```python
from build123d import *

# Parameters (mm, degrees)
SKETCH1_W           = 24.54
SKETCH1_H           = 35.2
MAIN_BODY_DEPTH     = 35.2
SKETCH2_R           = 11
LIP_DEPTH           = 2.25
SKETCH3_R           = 2.5
SHAFT_DEPTH         = 14
CHAMFER1_SIZE       = 5
SKETCH4_R           = 1.5
BOSS_EXTRUDE4_DEPTH = 6


with BuildPart() as part:
    # Sketch1 → Main body (new body)
    with BuildSketch(Plane(origin=(0, 0, 0), x_dir=(1, 0, 0), z_dir=(0, 1, 0))):
        with Locations((12.27, 17.6)):
            Rectangle(SKETCH1_W, SKETCH1_H)
    extrude(amount=MAIN_BODY_DEPTH)

    # Sketch2 → lip (add)
    with BuildSketch(Plane(origin=(24.54, 0, 0), x_dir=(0, 0, -1), z_dir=(1, 0, 0))):
        with Locations((17.6, 17.6)):
            Circle(SKETCH2_R)
    extrude(amount=LIP_DEPTH)

    # Sketch3 → shaft (add)
    with BuildSketch(Plane(origin=(26.79, 0, 0), x_dir=(0, 0, -1), z_dir=(1, 0, 0))):
        with Locations((17.6, 17.6)):
            Circle(SKETCH3_R)
    extrude(amount=SHAFT_DEPTH)

    # Chamfer1
    chamfer1_edges = [part.edges().sort_by_distance(p)[0] for p in [
        (12.27, 35.2, -35.2),
        (12.27, 0, -35.2),
        (12.27, 0, 0),
        (12.27, 35.2, 0),
    ]]
    chamfer(chamfer1_edges, length=CHAMFER1_SIZE)

    # Sketch4 → Boss-Extrude4 (add)
    with BuildSketch(Plane(origin=(24.54, 0, 0), x_dir=(0, 0, -1), z_dir=(1, 0, 0))):
        with Locations((30.6, 30.6)):
            Circle(SKETCH4_R)
        with Locations((30.6, 4.6)):
            Circle(SKETCH4_R)
        with Locations((4.6, 30.6)):
            Circle(SKETCH4_R)
        with Locations((4.6, 4.6)):
            Circle(SKETCH4_R)
    extrude(amount=BOSS_EXTRUDE4_DEPTH)


solid = part.part
```
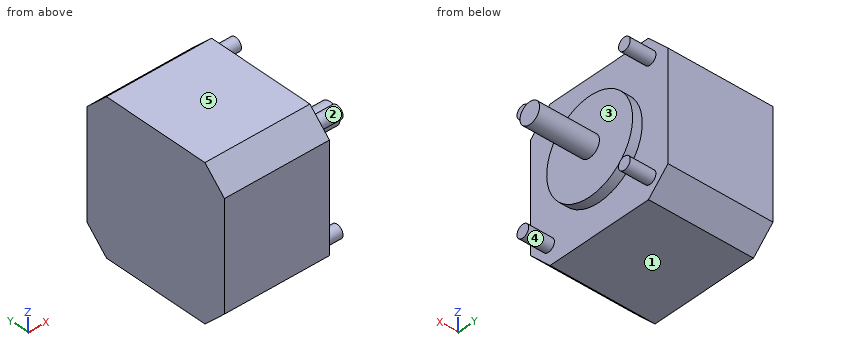
CAD build for the part. Positions are in the model's coordinates, mm. Face numbers are marked on the shaded views. A direction names the side the tool comes from. Round coordinates to 2 decimals unless told otherwise and drop trailing zeros. Write each loop counter-clockwise with the first axis right and the second up, starting at its lowest first coordinate (ties: lowest second). Pieces come first, ordered by that corner, then holes. Notation, with made-up numbers: (48.5, 49) - (94.5, 49) arc R14 ccw to (94.5, 76) - close; hole circle Ø2 at (70.25, -11.5). An arc over 180 degrees is marked (long way). Return JSON: item names as keys, results as strings. Group by question number.
Item 1: Band-saw the part on B-B on y = 17.6. List the corners of the cut face in (x, z).
Item 2: Mould opens along Z. For the marked faces 1, 2 and 3 say: +Z half, -Z half, draft (parallel to the pull), parting line (faces both ways), or undercut.
Item 3: Band-saw the part on C-C on z = -17.6. List the corners of the cut face in (x, y).
Item 4: Band-saw the part on D-D on z = -2.5. List the corners of the cut face in (x, y).
Item 5: 3-axis set-ups, long thin cutter, end or side, ignore diameter. For the marked faces 4 and 5: which of +Z, -Z, +X, -X, +Y, -Y reach the whole face in a straight line?
Item 6: Band-saw the part on A-A on x = 16. List the corners of the cut face in (y, z), plus the area to 3 significant figures.
Item 7: Flat gauge pins, fed straight in: pin 1 Ø2.5 at (y, z) = (30.5, -31) entering from +X; pin 2 Ø8 at (x, y) = (34, 13.5) entering from +Z; pin 3 Ø2 at (x, z) = (26, -6) entering from -Y. Where does each tip first touch, or does it go through?
Item 8: Probe probe 1 along X at (y, z) = (21, -32.5); probe 2 along Y at (x, z) = (25.5, -31.5); probe 3 along X at (y, z) = (11, -16). List the from-to ranges inside material, lowest first.
Resolved:
{
 "1": {"outline": "(0, -35.2) - (24.54, -35.2) - (24.54, -28.6) - (26.79, -28.6) - (26.79, -20.1) - (40.79, -20.1) - (40.79, -15.1) - (26.79, -15.1) - (26.79, -6.6) - (24.54, -6.6) - (24.54, 0) - (0, 0) - close"},
 "2": {"face 1": "-Z half", "face 2": "undercut", "face 3": "draft"},
 "3": {"outline": "(0, 0) - (24.54, 0) - (24.54, 6.6) - (26.79, 6.6) - (26.79, 15.1) - (40.79, 15.1) - (40.79, 20.1) - (26.79, 20.1) - (26.79, 28.6) - (24.54, 28.6) - (24.54, 35.2) - (0, 35.2) - close"},
 "4": {"outline": "(0, 2.5) - (24.54, 2.5) - (24.54, 32.7) - (0, 32.7) - close"},
 "5": {"face 4": "+X", "face 5": "+Z, +X, -X, +Y, -Y"},
 "6": {"outline": "(0, -30.2) - (5, -35.2) - (30.2, -35.2) - (35.2, -30.2) - (35.2, -5) - (30.2, 0) - (5, 0) - (0, -5) - close", "area": "1,190 mm²"},
 "7": {"pin 1": "stops at x = 30.54", "pin 2": "stops at z = -15.1", "pin 3": "stops at y = 3.15"},
 "8": {"probe 1": "x = 0 to 24.54", "probe 2": "y = 3.4 to 5.8, 29.4 to 31.8", "probe 3": "x = 0 to 26.79"}
}
